The model under review builds one solid part; all positions refer to its coordinate system, in mm. Face numbers are marked on the shaded views. Round coordinates to 2 decimals unless told otherwise and drop trailing zeros. Loops run counter-clockwise (first coordinate to the right, second up) from the corner with the lowest first, then second, coordinate; pieces in that order, holes last. Notation, with made-up numbers: (-29, -7) - (7, -7) arc R14 ccw to (7, 9) - close; hole circle Ø3 at (2.5, 18.25). An arc over 180 degrees is marked (long way). Answer as CSV lines item,"result".
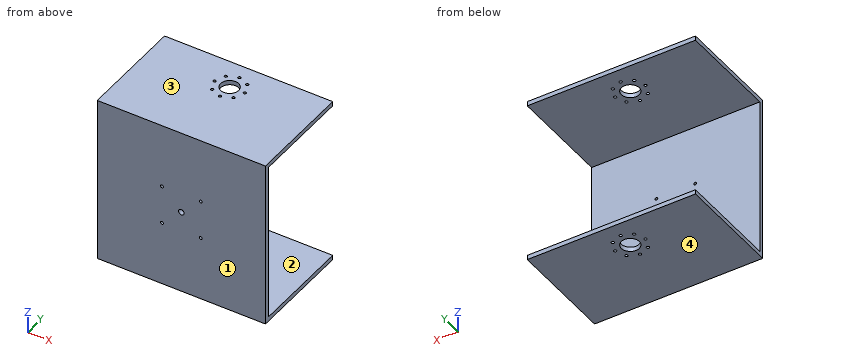
from build123d import *

# Parameters (mm, degrees)
SKETCH5_W           = 300
SKETCH5_H           = 300
BOSS_EXTRUDE4_DEPTH = 8
SKETCH6_R           = 5
SKETCH6_R_2         = 2.5
CUT_EXTRUDE2_DEPTH  = 16
SKETCH7_W           = 300
SKETCH7_H           = 8
BOSS_EXTRUDE5_DEPTH = 180
SKETCH9_R           = 16
CUT_EXTRUDE3_DEPTH  = 350
SKETCH11_R          = 2.5
CUT_EXTRUDE4_DEPTH  = 310


with BuildPart() as part:
    # Sketch5 → Boss-Extrude4 (new body)
    with BuildSketch(Plane(origin=(0, 0, 0), x_dir=(1, 0, 0), z_dir=(0, 1, 0))):
        Rectangle(SKETCH5_W, SKETCH5_H)
    extrude(amount=BOSS_EXTRUDE4_DEPTH)

    # Sketch6 → Cut-Extrude2 (cut)
    with BuildSketch(Plane(origin=(0, 8, 0), x_dir=(1, 0, 0), z_dir=(0, 1, 0))):
        with Locations(Location((0, 0, 0), (0, 0, 270))):
            Circle(SKETCH6_R)
        with Locations(Location((-34.62667873, 34.62667873, 0), (0, 0, 270))):
            Circle(SKETCH6_R_2)
        with Locations(Location((34.62667873, 34.62667873, 0), (0, 0, 270))):
            Circle(SKETCH6_R_2)
        with Locations(Location((34.62667873, -34.62667873, 0), (0, 0, 270))):
            Circle(SKETCH6_R_2)
        with Locations(Location((-34.62667873, -34.62667873, 0), (0, 0, 270))):
            Circle(SKETCH6_R_2)
    extrude(amount=-CUT_EXTRUDE2_DEPTH, mode=Mode.SUBTRACT)

    # Sketch7 → Boss-Extrude5 (add)
    with BuildSketch(Plane(origin=(0, 8, 0), x_dir=(1, 0, 0), z_dir=(0, 1, 0))):
        with Locations((0, 146)):
            Rectangle(SKETCH7_W, SKETCH7_H)
        with Locations((0, -146)):
            Rectangle(SKETCH7_W, SKETCH7_H)
    extrude(amount=BOSS_EXTRUDE5_DEPTH)

    # Sketch9 → Cut-Extrude3 (cut)
    with BuildSketch(Plane.XY.offset(150)):
        with Locations((0, 135)):
            Circle(SKETCH9_R)
    extrude(amount=-CUT_EXTRUDE3_DEPTH, mode=Mode.SUBTRACT)

    # Sketch11 → Cut-Extrude4 (cut)
    with BuildSketch(Plane.XY.offset(150)):
        with Locations((0, 162)):
            Circle(SKETCH11_R)
        with Locations((19.091883092, 154.091883092)):
            Circle(SKETCH11_R)
        with Locations((27, 135)):
            Circle(SKETCH11_R)
        with Locations((19.091883092, 115.908116908)):
            Circle(SKETCH11_R)
        with Locations((0, 108)):
            Circle(SKETCH11_R)
        with Locations((-19.091883092, 115.908116908)):
            Circle(SKETCH11_R)
        with Locations((-27, 135)):
            Circle(SKETCH11_R)
        with Locations((-19.091883092, 154.091883092)):
            Circle(SKETCH11_R)
    extrude(amount=-CUT_EXTRUDE4_DEPTH, mode=Mode.SUBTRACT)


solid = part.part
1. Clearance check with a flat-ended pin moving along its axis: pin 1 (3 mm diameter, centred on x = 34.63, z = -34.63, fed in from +Y). State where the tip first meets the part, or that it passes through.
Numbers:
pin 1,"passes through"
2. Take a section at B-B (z = -82.5). State the section outline as (x, y) points.
Numbers:
outline,"(-150, 0) - (150, 0) - (150, 8) - (-150, 8) - close"
3. Take a section at A-A (x = 110.5). State the section outline as (y, z) points.
Numbers:
outline,"(0, -150) - (188, -150) - (188, -142) - (8, -142) - (8, 142) - (188, 142) - (188, 150) - (0, 150) - close"
4. Wall thickness on probe 1 along Z at (x, y) = (-37.5, 91); probe 2 along Y at (x, z) = (27, -145); probe 3 along Y at (x, z) = (132.5, -35): over which ranges is each line inside the solid? List them lowest first.
Numbers:
probe 1,"z = -150 to -142, 142 to 150"
probe 2,"y = 0 to 132.5, 137.5 to 188"
probe 3,"y = 0 to 8"
5. Draft analysis for pull direction Z (two halves, no side actions). For the marked faces 1, 2, 3 and 4, state which applies: +Z half, -Z half, draft (parallel to the pull), parting line (faces both ways), or undercut.
Numbers:
face 1,"draft"
face 2,"undercut"
face 3,"+Z half"
face 4,"-Z half"
